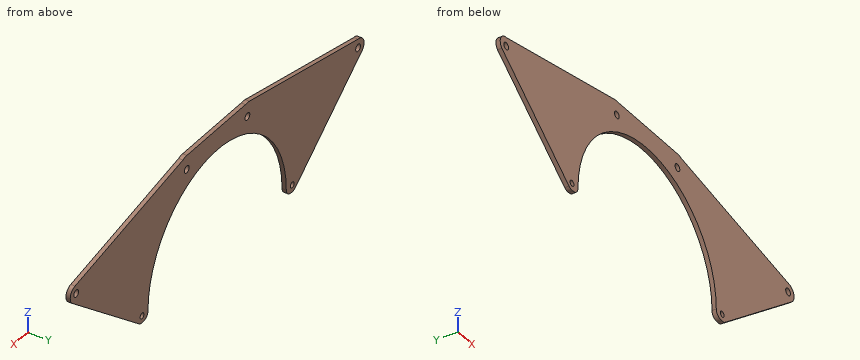
```python
from build123d import *

# Parameters (mm, degrees)
F0_R     = 4
F0_R_2   = 5
F1_DEPTH = 6
F2_R     = 10


with BuildPart() as f1:
    # F0 (on Front) → F1 (new body)
    with BuildSketch(Plane.XZ):
        with BuildLine():
            ThreePointArc((-144.660726, -9.91334), (-0.357114, 144.99956), (144.707801, -9.200666))
            Line((144.707801, -9.200666), (156.522168, -9.952077))
            Line((156.522168, -9.952077), (157.209119, -9.995769))
            ThreePointArc((157.209119, -9.995769), (160.702353, -9.47338), (163.796076, -7.769133))
            Line((163.796076, -7.769133), (302.56026, 104.68483))
            Line((302.56026, 104.68483), (304.128535, 105.955755))
            ThreePointArc((304.128535, 105.955755), (307.51077, 118.462861), (297.98923, 127.249642))
            Line((297.98923, 127.249642), (71.733118, 173.226787))
            ThreePointArc((71.733118, 173.226787), (67.679112, 174.558503), (63.434867, 174.999894))
            Line((63.434867, 174.999894), (-59.51749, 174.59948))
            ThreePointArc((-59.51749, 174.59948), (-63.53231, 174.999974), (-67.545815, 174.58651))
            Line((-67.545815, 174.58651), (-295.5, 127.5))
            ThreePointArc((-295.5, 127.5), (-306.963068, 119.984783), (-304.642546, 106.47569))
            Line((-304.642546, 106.47569), (-163.799516, -7.766344))
            ThreePointArc((-163.799516, -7.766344), (-161.469112, -9.17857), (-158.843996, -9.909272))
            Line((-158.843996, -9.909272), (-156.161689, -9.910041))
            Line((-156.161689, -9.910041), (-144.660726, -9.91334))
        make_face()
        with Locations((-157.5, 0)):
            Circle(F0_R, mode=Mode.SUBTRACT)
        with Locations((157.5, 0)):
            Circle(F0_R, mode=Mode.SUBTRACT)
        with Locations((-295.5, 115)):
            Circle(F0_R_2, mode=Mode.SUBTRACT)
        with Locations((-63.5, 155)):
            Circle(F0_R_2, mode=Mode.SUBTRACT)
        with Locations((295.5, 115)):
            Circle(F0_R_2, mode=Mode.SUBTRACT)
        with Locations((63.5, 155)):
            Circle(F0_R_2, mode=Mode.SUBTRACT)
        with BuildLine():
            Line((157.209119, -9.995769), (156.522168, -9.952077))
            ThreePointArc((156.522168, -9.952077), (156.865267, -9.979835), (157.209119, -9.995769))
        make_face()
        with BuildLine():
            ThreePointArc((-158.843996, -9.909272), (-157.502868, -10), (-156.161689, -9.910041))
            Line((-156.161689, -9.910041), (-158.843996, -9.909272))
        make_face()
        with BuildLine():
            Line((304.128535, 105.955755), (302.56026, 104.68483))
            ThreePointArc((302.56026, 104.68483), (303.370095, 105.288584), (304.128535, 105.955755))
        make_face()
    extrude(amount=F1_DEPTH)

    # F2
    f2_edges = [f1.edges().sort_by_distance(p)[0] for p in [
        (-144.660726, -3, -9.91334),
        (144.707801, -3, -9.200666),
    ]]
    fillet(f2_edges, radius=F2_R)


solid = f1.part
```
Source: CAD feature listing. Evaluate the final solid. Frame: model axes, mm. Give positions to 0.01 mm unless a question says otherwise; leave off trailing zeros. Loops run counter-clockwise (first coordinate to the right, second up) from the corner with the lowest first, then second, coordinate; pieces in that order, holes last. Notation, with made-up numbers: M -18,22 L 10,22 A11 ccw 10,34 Z; hole C 65,37 d5. An arc over 180 degrees is marked long. Put each result on its own line as item: value.
Q1. Section B-B (x = -219). Return the cut outline in (y, z).
Response values:
outline: M -6,37.01 L 0,37.01 L 0,143.3 L -6,143.3 Z
Q2. Section A-A (z = 42). Return the cut outline in (x, y), and give its area (3 significant figures).
Response values:
outline: M -225.15,-6 L -138.78,-6 L -138.78,0 L -225.15,0 Z; M 138.78,-6 L 225.21,-6 L 225.21,0 L 138.78,0 Z
area: 1,040 mm²
Q3. Line query: probe 1 along Z at (x, y) = (63.5, -1.9); probe 2 along Z at (x, y) = (-295.5, -2.7); probe 3 along X at (y, z) = (-5.45, 107). Output: solid intervals per line, ascending. Write a range as [from, to].
Response values:
probe 1: z = [130.36, 150], [160, 175]
probe 2: z = [99.06, 110], [120, 127.5]
probe 3: x = [-305.1, -97.86], [97.86, 305.1]
Q4. Section C-C (x = 0). Return the cut outline in (y, z), and give its area (3 significant figures).
Response values:
outline: M -6,145 L 0,145 L 0,174.79 L -6,174.79 Z
area: 179 mm²
Q5. Pin query (flat end, axial travel): P1, Ø1.3, axis at x = -155.5, y = -4.5, coming from the -Z side; P2, Ø13, axis at x = -157.5, z = 0, coming from the -Y side; P3, Ø1, axis at x = -180, y = -5, coming from the -Z side; P4, Ø8, axis at x = -295.5, z = 115, coming from the +Y side. Return the tip coordinate at first contact, or that it passes through.
Response values:
P1: stops at z = -9.91
P2: stops at y = -6
P3: stops at z = 4.97
P4: passes through
